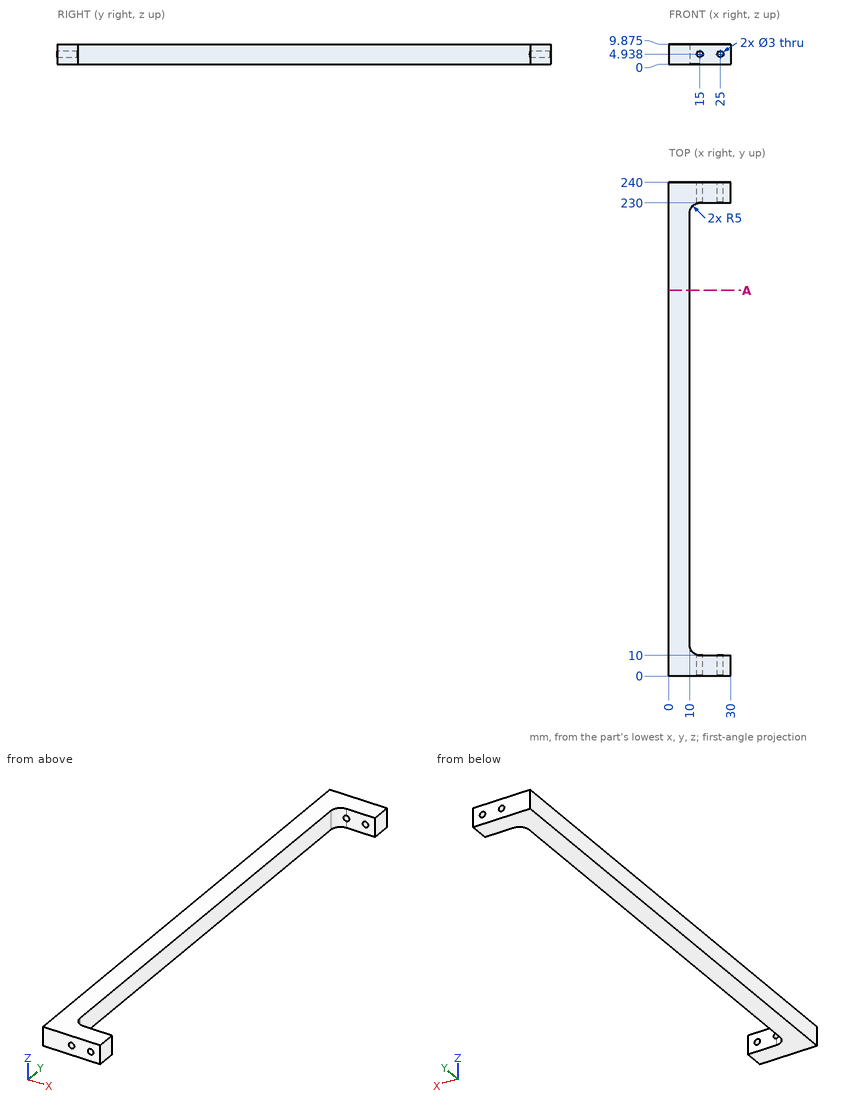
Check sheet for the drawn part. Datum: minimum x, y, z corner. Units: mm. Coordinates: 2 decimals unless noted, no trailing zeros. Loops run counter-clockwise (first coordinate to the right, second up) from the corner with the lowest first, then second, coordinate; pieces in that order, holes last. Notation, with made-up numbers: (-40, 26.5) -> (8, 26.5) arc R23 ccw to (8, 36.5) -> close; hole circle Ø2 at (47, 88.5). An arc over 180 degrees is marked (long way). Answer as CSV lines item,"result".
1) Thickness scan on L1, parallel to Z at x = 15, y = 235 (1 decimal); L2, parallel to Y at x = 20, z = 3.25; L3, parallel to X at y = 164.5, z = 7.75. Record the ranges inside material, lowest first. Write a range as from..to.
Found:
L1,"z = 0..3.4, 6.4..9.9"
L2,"y = 0..10, 230..240"
L3,"x = 0..10"
2) Cross-section at A-A, the plane y = 187.5. Record the cut outline in (x, z) (1 decimal).
Found:
outline,"(0, 0) -> (10, 0) -> (10, 9.9) -> (0, 9.9) -> close"
3) Depth check by flat-ended pin: pin 1 (1.8 mm diameter, centred on x = 25, z = 4.94, fed in from -Y); pin 2 (5 mm diameter, centred on y = 123.5, z = 7, fed in from +X). Enter the tip coordinate at first touch or a pass-through.
Found:
pin 1,"passes through"
pin 2,"stops at x = 10"
